Answer from the drawing. Dimensions are ordinates in mm from the lowest x, y and z of the part. Round coordinates to 2 decimals unless told otherwise and drop trailing zeros. Loops run counter-clockwise (first coordinate to the right, second up) from the corner with the lowest first, then second, coordinate; pieces in that order, holes last. Notation, with made-up numbers: (-0.75, -15.5) -> (38.25, -15.5) arc R25 cw to (38.25, 1.5) -> close; hole circle Ø8 at (84, -1). An arc over 180 degrees is marked (long way). One line per question, with ' | ' between items.
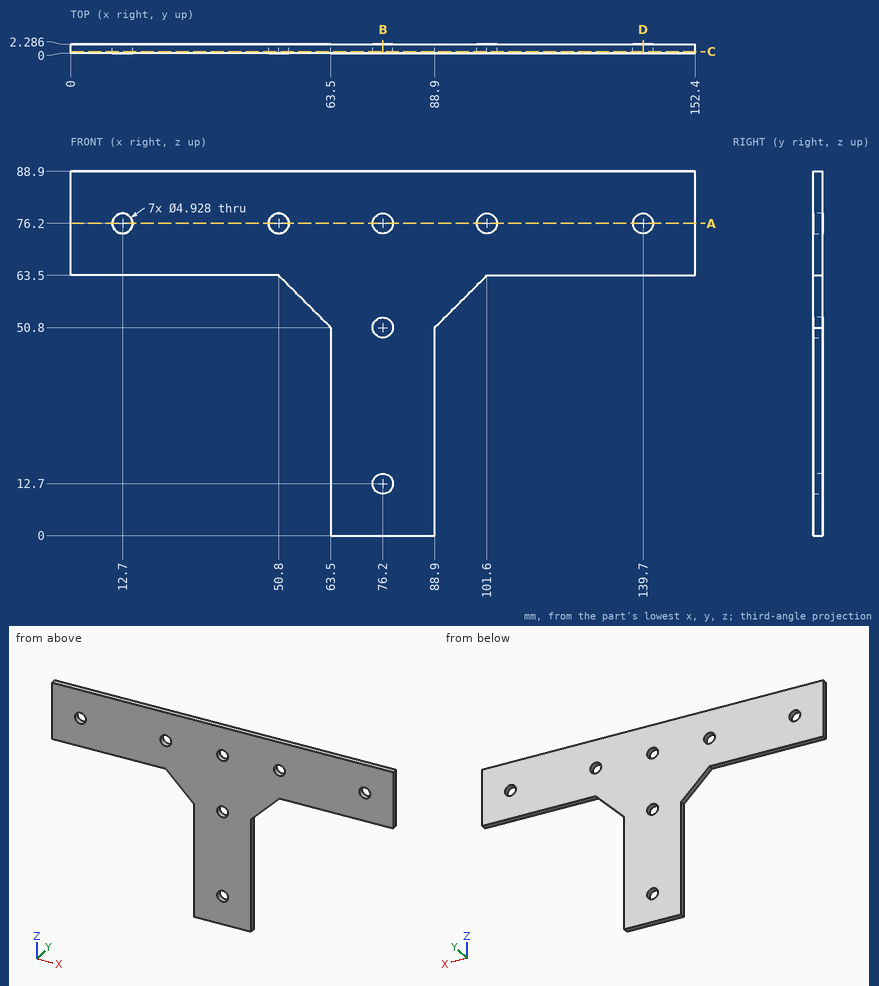
Q1. A cutting plane is placed at A-A on z = 76.2. Give the vertices of the cut face in (x, y), plus the area to 3 significant figures.
Numbers:
outline: (0, 0) -> (10.24, 0) -> (10.24, 2.29) -> (0, 2.29) -> close; (15.16, 0) -> (48.34, 0) -> (48.34, 2.29) -> (15.16, 2.29) -> close; (53.26, 0) -> (73.74, 0) -> (73.74, 2.29) -> (53.26, 2.29) -> close; (78.66, 0) -> (99.14, 0) -> (99.14, 2.29) -> (78.66, 2.29) -> close; (104.06, 0) -> (137.24, 0) -> (137.24, 2.29) -> (104.06, 2.29) -> close; (142.16, 0) -> (152.4, 0) -> (152.4, 2.29) -> (142.16, 2.29) -> close | area: 292 mm^2
Q2. A cutting plane is placed at C-C on y = 0.45. Give the vertices of the cut face in (x, z), plus the area to 3 significant figures.
Numbers:
outline: (0, 63.5) -> (50.8, 63.5) -> (63.5, 50.8) -> (63.5, 0) -> (88.9, 0) -> (88.9, 50.8) -> (101.6, 63.5) -> (152.4, 63.5) -> (152.4, 88.9) -> (0, 88.9) -> close; hole circle Ø4.93 at (12.7, 76.2); hole circle Ø4.93 at (50.8, 76.2); hole circle Ø4.93 at (76.2, 12.7); hole circle Ø4.93 at (76.2, 50.8); hole circle Ø4.93 at (76.2, 76.2); hole circle Ø4.93 at (101.6, 76.2); hole circle Ø4.93 at (139.7, 76.2) | area: 5,510 mm^2
Q3. A cutting plane is placed at D-D on x = 139.7. Give the vertices of the cut face in (y, z), plus the area to 3 significant figures.
Numbers:
outline: (0, 63.5) -> (2.29, 63.5) -> (2.29, 73.74) -> (0, 73.74) -> close; (0, 78.66) -> (2.29, 78.66) -> (2.29, 88.9) -> (0, 88.9) -> close | area: 46.8 mm^2
Q4. A cutting plane is placed at B-B on x = 76.2. Give the vertices of the cut face in (y, z).
Numbers:
outline: (0, 0) -> (2.29, 0) -> (2.29, 10.24) -> (0, 10.24) -> close; (0, 15.16) -> (2.29, 15.16) -> (2.29, 48.34) -> (0, 48.34) -> close; (0, 53.26) -> (2.29, 53.26) -> (2.29, 73.74) -> (0, 73.74) -> close; (0, 78.66) -> (2.29, 78.66) -> (2.29, 88.9) -> (0, 88.9) -> close
Q5. Find the intervals of material crossed by line 1 (X direction, y = 1.7, z = 76.2); line 2 (X direction, y = 1.75, z = 12.7); line 3 (Z direction, x = 26, y = 0.7), in increasing order. Write a range as from..to.
Numbers:
line 1: 0..10.24, 15.16..48.34, 53.26..73.74, 78.66..99.14, 104.06..137.24, 142.16..152.4 | line 2: 63.5..73.74, 78.66..88.9 | line 3: 63.5..88.9
Q6. Given pin 1 Ø1.1 at (x, y) = (131, 1) entering from -Z, flat-ended and moving along its own axis, determine where the tip first touches the part or whether it passes through.
Numbers:
pin 1: z = 63.5
